CAD build for the part. Positions are in the model's coordinates, mm. A direction names the side the tool comes from. Coordinates: 2 decimals unless noted, no trailing zeros. Loops run counter-clockwise (first coordinate to the right, second up) from the corner with the lowest first, then second, coordinate; pieces in that order, holes last.
1) Wall check: line 1 along Y through (x, z) = (30, -2); line 2 along Y through (x, z) = (-5.5, 0); line 3 along Z through (x, y) = (-5, 1.75). Give the ranges that are in metal, low to high.
2) Pin check, flat tips, straight feed: pin 1 Ø0.8 at (y, z) = (2, -2) entering from -X; pin 2 Ø0.8 at (y, z) = (0.5, 2.5) entering from -X; pin 3 Ø1.5 at (x, y) = (4.5, -0.5) entering from -Z. Stop position of each tip, or through.
3) Which spindle directions (+Z, -Z, +X, -X, +Y, -Y) get a long thin tool onto all of the face, cutting with end or side? Do faces 1 (the flat face through (-3.3, -3.2, 0)), 2 (the cylindrical face through (20.394, -3.905, -0.867)), 3 (the flat face through (40, 0, 0)). Say none if no direction does.
4) Saw through at A-A, the plane x = -4.5. Write the cut outline in (y, z).
5) Two-plate mould, pull along Z, no slides. Class faces 4 (the flat face through (-3.3, 1.59, -2.75)), 5 (the cylindrical face through (-3.55, -3.955, -5.158)), 6 (the flat face through (0, -4, 3)): +Z half, -Z half, draft (parallel to the pull), parting line (faces both ways), or undercut.
6) Saw through at B-B, the plane x = 23. Write the cut outline in (y, z), and give its area (3 significant figures).
```python
from build123d import *

# Parameters (mm, degrees)
ENL_V_MAT_EXTRU_1_DEPTH = 8
ESQUISSE3_R             = 4.875
BOSS_EXTRU_1_DEPTH      = 4.161898962


with BuildPart() as part:
    # Esquisse1 → Révolution1 (revolve)
    with BuildSketch(Plane(origin=(0, 0, 0), x_dir=(1, 0, 0), z_dir=(0, 1, 0)), mode=Mode.PRIVATE) as r_volution1_sk:
        with BuildLine():
            Line((-1.567949192, 0), (-3.3, 3))
            Line((-3.3, 3), (-7.57, 3))
            Line((-7.57, 3), (-8, 3.43))
            Line((-8, 3.43), (-8, 5.7))
            ThreePointArc((-8, 5.7), (-7.765685425, 6.265685425), (-7.2, 6.5))
            Line((-7.2, 6.5), (0, 6.5))
            Line((0, 6.5), (0, 4.6))
            ThreePointArc((0, 4.6), (0.076642269, 4.36454347), (0.277198888, 4.219316553))
            Line((0.277198888, 4.219316553), (0.897198888, 4.019316553))
            ThreePointArc((0.897198888, 4.019316553), (0.957844465, 4.004858646), (1.02, 4))
            Line((1.02, 4), (39.233, 4))
            Line((39.233, 4), (40, 3.233))
            Line((40, 3.233), (40, 0))
            Line((40, 0), (-1.567949192, 0))
        make_face()
    revolve(r_volution1_sk.sketch.rotate(Axis((43, 0, 0), (-1, 0, 0)), 180), axis=Axis((43, 0, 0), (-1, 0, 0)))

    # Esquisse2 → Enlèv. mat.-Extru.1 (cut)
    with BuildSketch(Plane(origin=(-3.3, 0, 0), x_dir=(0, 0, -1), z_dir=(1, 0, 0))):
        Polygon((-3, 1.732050808), (-3, -1.732050808), (0, -3.464101615), (3, -1.732050808), (3, 1.732050808), (0, 3.464101615), align=None)
    extrude(amount=-ENL_V_MAT_EXTRU_1_DEPTH, mode=Mode.SUBTRACT)


with BuildPart() as body_2:
    # Esquisse3 → Boss.-Extru.1 (new body)
    with BuildSketch(Plane(origin=(0, 0, 0), x_dir=(0, 0, -1), z_dir=(1, 0, 0))):
        Circle(ESQUISSE3_R)
    extrude(amount=-BOSS_EXTRU_1_DEPTH)

    # SupprimerFace1: 1 face struck out; the rest of the skin is kept as a surface, the solid goes
    supprimerface1_1_drop = [body_2.part.faces().sort_by_distance(Vector(p))[0] for p in ((-4.161898962, 0, 0),)]
    supprimerface1_1 = Shell(body_2.part.faces() - supprimerface1_1_drop)


solid = part.part
```
Data:
1. line 1: y = -3.46 to 3.46
1. line 2: y = -6.5 to -3.46, 3.46 to 6.5
1. line 3: z = -6.26 to -2.97, 2.97 to 6.26
2. pin 1: stops at x = -7.8
2. pin 2: stops at x = -3.27
2. pin 3: stops at z = -4
3. face 1: -X
3. face 2: +X
3. face 3: +Z, -Z, +X, +Y, -Y
4. outline: circle Ø13 at (0, 0); hole (-3.46, 0) - (-1.73, -3) - (1.73, -3) - (3.46, 0) - (1.73, 3) - (-1.73, 3) - close
5. face 4: undercut
5. face 5: parting line
5. face 6: draft
6. outline: circle Ø8 at (0, 0)
6. area: 50.3 mm2
